Design review of the part built by this model. Coordinates are the model's own, in mm. A direction names the side the tool comes from. Round coordinates to 2 decimals unless told otherwise and drop trailing zeros. Order: outer loops, then holes, each group sorted by start corner. A loop starts at its lowest first (then second) coordinate and runs counter-clockwise, first axis right, second up. Notation, with made-up numbers: (73.25, 12) - (112.25, 12) arc R16 cw to (112.25, 36) - close; hole circle Ø5 at (-3.75, 1.5). An arc over 180 degrees is marked (long way). Write item = value, one per line.
from build123d import *

# Parameters (mm, degrees)
BOSS_EXTRUDE1_DEPTH      = 15.6
BOSS_EXTRUDE1_DEPTH_BACK = 15.6
SKETCH1_R                = 2
BOSS_EXTRUDE2_DEPTH      = 5
BOSS_EXTRUDE2_DEPTH_BACK = 5
SKETCH3_W                = 10
SKETCH3_H                = 5


with BuildPart() as part:
    # Sketch1 → Boss-Extrude1 (new, two sides: drawn at the far end of the back side and taken through both)
    with BuildSketch(Plane(origin=(0, 0, 0), x_dir=(1, 0, 0), z_dir=(0, 1, 0)).offset(-BOSS_EXTRUDE1_DEPTH_BACK)):
        with Locations(Location((0, 0, 0), (0, 0, 270))):
            Circle(SKETCH1_R)
    extrude(amount=BOSS_EXTRUDE1_DEPTH + BOSS_EXTRUDE1_DEPTH_BACK)

    # Sketch3 → Boss-Extrude2 (add, two sides: drawn at the far end of the back side and taken through both)
    with BuildSketch(Plane(origin=(0, 0, 0), x_dir=(0, 0, -1), z_dir=(1, 0, 0)).offset(-BOSS_EXTRUDE2_DEPTH_BACK)):
        with Locations((0, -5)):
            Rectangle(SKETCH3_W, SKETCH3_H)
    extrude(amount=BOSS_EXTRUDE2_DEPTH + BOSS_EXTRUDE2_DEPTH_BACK)


solid = part.part
1) We need section C-C on y = -1. Write out the cut boundary in (x, z), and give its area (3 significant figures).
Findings:
outline = circle Ø4 at (0, 0)
area = 12.6 mm^2
2) For faces 1 (the flat face through (0, -5, -5)), 2 (the cylindrical face through (-2, 6, 0)), 3 (the cylindrical face through (-2, -12, 0)), list the 3-axis set-ups (+Z, -Z, +X, -X, +Y, -Y) from which the entire face can be reached by the end or side of a thin tool; tool diameter is ignored.
Findings:
face_1 = -Z, +X, -X, +Y, -Y
face_2 = +Y
face_3 = -Y
3) We need section D-D on z = -2.75. Write out the cut boundary in (x, y).
Findings:
outline = (-5, -7.5) - (5, -7.5) - (5, -2.5) - (-5, -2.5) - close
4) We need section A-A on x = 0. Write out the cut boundary in (y, z).
Findings:
outline = (-15.6, -2) - (-7.5, -2) - (-7.5, -5) - (-2.5, -5) - (-2.5, -2) - (15.6, -2) - (15.6, 2) - (-2.5, 2) - (-2.5, 5) - (-7.5, 5) - (-7.5, 2) - (-15.6, 2) - close
5) We need section B-B on z = 0. Write out the cut boundary in (x, y).
Findings:
outline = (-5, -7.5) - (-2, -7.5) - (-2, -15.6) - (2, -15.6) - (2, -7.5) - (5, -7.5) - (5, -2.5) - (2, -2.5) - (2, 15.6) - (-2, 15.6) - (-2, -2.5) - (-5, -2.5) - close
6) Clearance check with flat-ended pins moving along their axes: pin 1 Ø2 at (x, z) = (-1, -3) entering from -Y; pin 2 Ø1 at (x, z) = (3, 0) entering from +Y; pin 3 Ø3 at (x, z) = (-2, 2) entering from -Y. State where each tip first meets the part, or that it passes through.
Findings:
pin_1 = -7.5
pin_2 = -2.5
pin_3 = -15.6
7) To check wall thickness, follow L1, parallel to Y at x = 0, z = 2.5; L2, parallel to X at y = 9.5, z = 0; L3, parallel to Z at x = -0.25, y = -9. State the ranges of each line that lie inside material, in increasing order. Write a range as from..to.
Findings:
L1 = -7.5..-2.5
L2 = -2..2
L3 = -1.98..1.98
